```python
from build123d import *

# Parameters (mm, degrees)
BOSS_EXTRUDE1_DEPTH = 70
SKETCH3_R           = 1.5
SKETCH3_W           = 20
SKETCH3_H           = 41
CUT_EXTRUDE1_DEPTH  = 50


with BuildPart() as part:
    # Sketch2 → Boss-Extrude1 (new body)
    with BuildSketch(Plane(origin=(0, 0, 0), x_dir=(1, 0, 0), z_dir=(0, 1, 0))):
        with BuildLine():
            ThreePointArc((6, -69), (2.485281374, -77.485281374), (-6, -81))
            Line((-6, -81), (-35, -81))
            Line((-35, -81), (-35, -75))
            Line((-35, -75), (-6, -75))
            ThreePointArc((-6, -75), (-1.757359313, -73.242640687), (0, -69))
            Line((0, -69), (0, 0))
            Line((0, 0), (6, 0))
            Line((6, 0), (6, -69))
        make_face()
    extrude(amount=BOSS_EXTRUDE1_DEPTH)

    # Sketch3 → Cut-Extrude1 (cut)
    with BuildSketch(Plane.XY.offset(81)):
        with Locations((-19, 60)):
            Circle(SKETCH3_R)
        with Locations((-13, 60)):
            Circle(SKETCH3_R)
        with Locations((-13, 10)):
            Circle(SKETCH3_R)
        with Locations((-19, 10)):
            Circle(SKETCH3_R)
        with Locations((-16, 35)):
            Rectangle(SKETCH3_W, SKETCH3_H)
    extrude(amount=-CUT_EXTRUDE1_DEPTH, mode=Mode.SUBTRACT)


solid = part.part
```
Check sheet for the modelled part. Datum: model origin and axes. Units: mm. A direction names the side the tool comes from. Give positions to 0.01 mm unless a question says otherwise; leave off trailing zeros. Order: outer loops, then holes, each group sorted by start corner. A loop starts at its lowest first (then second) coordinate and runs counter-clockwise, first axis right, second up. Notation, with made-up numbers: (65, 28) -> (94, 28) arc R23 ccw to (94, 53) -> close; hole circle Ø5 at (72.5, 82). An arc over 180 degrees is marked (long way). Return JSON: item names as keys, results as strings.
1. Cross-section at A-A, the plane x = -7. Record the cut outline in (y, z), plus the area to 3 significant figures.
From the geometry:
{"outline": "(0, 75) -> (14.5, 75) -> (14.5, 81) -> (0, 81) -> close; (55.5, 75) -> (70, 75) -> (70, 81) -> (55.5, 81) -> close", "area": "174 mm^2"}
2. Go/stop test with flat-tipped pins: P1, Ø23, axis at x = -15, y = 42.5, coming from the -Z side; P2, Ø2, axis at y = 53.5, z = 56, coming from the -X side; P3, Ø4, axis at x = -3.5, y = 32.5, coming from the +Z side. Record where each tip stops, or that it passes through.
From the geometry:
{"P1": "z = 74.45", "P2": "x = 0", "P3": "z = 80.99"}
3. Mould release check, pull along X, two halves, no side actions. Record for faces 1 (the flat face through (0, 35, 35)), 2 (the cylindrical face through (-14.2, 9.1, 78)), 3 (the flat face through (-27, 35, 75)): +X half, -X half, draft (parallel to the pull), parting line (faces both ways), or undercut.
From the geometry:
{"face 1": "-X half", "face 2": "undercut", "face 3": "draft"}
4. Cross-section at D-D, the plane y = 10. Record the cut outline in (x, z).
From the geometry:
{"outline": "(-35, 75) -> (-20.5, 75) -> (-20.5, 81) -> (-35, 81) -> close; (-17.5, 75) -> (-14.5, 75) -> (-14.5, 81) -> (-17.5, 81) -> close; (-11.5, 75) -> (-6, 75) arc R6 cw to (0, 69) -> (0, 0) -> (6, 0) -> (6, 69) arc R12 ccw to (-6, 81) -> (-11.5, 81) -> close"}
5. Cross-section at B-B, the plane y = 37. Record the cut outline in (x, z), plus the area to 3 significant figures.
From the geometry:
{"outline": "(-35, 75) -> (-26, 75) -> (-26, 81) -> (-35, 81) -> close; (-6, 75) arc R6 cw to (0, 69) -> (0, 0) -> (6, 0) -> (6, 69) arc R12 ccw to (-6, 81) -> close", "area": "553 mm^2"}
6. Set-up check for faces 4 (the cylindrical face through (2.58, 34.51, 77.39)), 5 (the flat face through (-6, 35, 78)): record each of +Z, -Z, +X, -X, +Y, -Y from which the full face is reachable in a straight line by a thin tool's end or side.
From the geometry:
{"face 4": "+Z, +X, +Y, -Y", "face 5": "+Z, -Z"}
7. Cross-section at C-C, the plane x = -19. Record the cut outline in (y, z).
From the geometry:
{"outline": "(0, 75) -> (8.5, 75) -> (8.5, 81) -> (0, 81) -> close; (11.5, 75) -> (14.5, 75) -> (14.5, 81) -> (11.5, 81) -> close; (55.5, 75) -> (58.5, 75) -> (58.5, 81) -> (55.5, 81) -> close; (61.5, 75) -> (70, 75) -> (70, 81) -> (61.5, 81) -> close"}
8. Material ranges on probe 1 along Y at (x, z) = (-13, 79); probe 2 along X at (y, z) = (33, 66); probe 3 along Z at (x, y) = (-23.5, 65.5), recorded low to high. Write a range as [from, to].
From the geometry:
{"probe 1": "[0, 8.5], [11.5, 14.5], [55.5, 58.5], [61.5, 70]", "probe 2": "[0, 6]", "probe 3": "[75, 81]"}
